```python
from build123d import *

# Parameters (mm, degrees)
F0_R     = 4
F1_DEPTH = 40
F2_R     = 6.5
F2_R_2   = 4
F3_DEPTH = 25
F4_R     = 2


with BuildPart() as f1:
    # F0 (on Front) → F1 (new body)
    with BuildSketch(Plane.XZ):
        with BuildLine():
            ThreePointArc((-8, 0), (0, -8), (8, 0))
            ThreePointArc((8, 0), (0, 8), (-8, 0))
        make_face()
        Circle(F0_R, mode=Mode.SUBTRACT)
        with BuildLine():
            Line((8, -10), (8, 0))
            ThreePointArc((8, 0), (0, -8), (-8, 0))
            Line((-8, 0), (-8, -10))
            Line((-8, -10), (8, -10))
        make_face()
    extrude(amount=F1_DEPTH)

    # F2 (on face) → F3 (cut)
    with BuildSketch(Plane.XZ.offset(40)):
        Circle(F2_R)
        Circle(F2_R_2, mode=Mode.SUBTRACT)
    extrude(amount=-F3_DEPTH, mode=Mode.SUBTRACT)

    # F4
    f4_edges = [f1.edges().sort_by_distance(p)[0] for p in [
        (0, -40, 8),
        (0, 0, 8),
    ]]
    fillet(f4_edges, radius=F4_R)


solid = f1.part
```
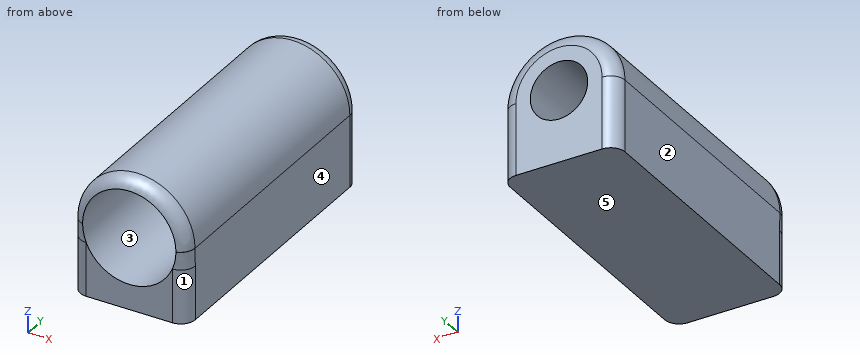
Read the model definition and answer for the solid it produces. Units are mm, in the model's axes. Face numbers are marked on the shaded views. A direction names the side the tool comes from. Round coordinates to 2 decimals unless told otherwise and drop trailing zeros. Write each loop counter-clockwise with the first axis right and the second up, starting at its lowest first coordinate (ties: lowest second). Pieces come first, ordered by that corner, then holes. Notation, with made-up numbers: (82, 6.25) - (120, 6.25) arc R12 ccw to (120, 10.25) - close; hole circle Ø1 at (17, 27.5). An arc over 180 degrees is marked (long way). One line per item, written item: value.
Q1. Straight lines are drawn through the part: line 1 (Z direction, x = 0, y = -4.75); line 2 (Z direction, x = 0, y = -26.5); line 3 (X direction, y = -22.75, z = 0). For each, find the intervals that lie inside material, in ascending order. Write a range as from..to.
The answers:
line 1: z = -10..-4, 4..8
line 2: z = -10..-6.5, 6.5..8
line 3: x = -8..-6.5, 6.5..8
Q2. For a pull along Z with two mould halves and no side action, classify the marked faces 3, 4 and 5 as pulls with the +Z half, pulls with the -Z half, needs draft (parallel to the pull), parting line crosses it, or undercut.
The answers:
face 3: undercut
face 4: needs draft
face 5: pulls with the -Z half
Q3. Each of these flat-tipped pins is pushed along its axis until it touches: P1, Ø2, axis at x = -4.5, y = -23.5, coming from the +Z side; P2, Ø5, axis at x = 0, z = 0, coming from the +Y side; P3, Ø3, axis at y = -17.5, z = 5.5, coming from the +X side; P4, Ø6.5, axis at x = -3, z = -0.5, coming from the -Y side. Where does it stop, or does it pass through?
The answers:
P1: stops at z = 7.19
P2: passes through
P3: stops at x = 6.93
P4: stops at y = -15
Q4. Which of the six approach directions +Z, -Z, +X, -X, +Y, -Y give full straight-line access (tool end or side, diameter ignored) to the marked faces 1 and 2?
The answers:
face 1: -Z, +X, -Y
face 2: +Z, -Z, -X, +Y, -Y
Q5. Find section B-B (y = -30.5). Determine the outline of the cut face in (x, z), and give its area (3 significant figures).
The answers:
outline: (-8, -10) - (8, -10) - (8, 0) arc R8 ccw to (-8, 0) - close; hole circle Ø13 at (0, 0)
area: 128 mm2
Q6. Find section A-A (y = -9). Determine the outline of the cut face in (x, z), and give its area (3 significant figures).
The answers:
outline: (-8, -10) - (8, -10) - (8, 0) arc R8 ccw to (-8, 0) - close; hole circle Ø8 at (0, 0)
area: 210 mm2
